from build123d import *

# Parameters (mm, degrees)
CROQUIS1_W               = 30
CROQUIS1_H               = 30
CROQUIS1_R               = 2.1
SALIENTE_EXTRUIR1_DEPTH  = 6
REDONDEO1_R              = 5
CROQUIS3_R               = 3.45
CORTAR_EXTRUIR2_DEPTH    = 2
REDONDEO1_OF_SIMETR_A1_R = 5
CROQUIS2_OUTSIDE_W       = 79.012
CROQUIS2_OUTSIDE_H       = 79.012
CROQUIS2_OUTSIDE_R       = 29
CORTAR_EXTRUIR1_DEPTH    = 3
CHAFL_N1_SIZE            = 0.5


with BuildPart() as part:
    # Croquis1 → Saliente-Extruir1 (new body)
    with BuildSketch(Plane(origin=(0, 0, 0), x_dir=(1, 0, 0), z_dir=(0, 1, 0))):
        with Locations((15, 15)):
            Rectangle(CROQUIS1_W, CROQUIS1_H)
        with Locations((25, 25)):
            Circle(CROQUIS1_R, mode=Mode.SUBTRACT)
        with BuildLine():
            Line((2.5, 3), (2.5, 25))
            ThreePointArc((2.5, 25), (4, 26.5), (5.5, 25))
            Line((5.5, 25), (5.5, 3))
            ThreePointArc((5.5, 3), (4, 1.5), (2.5, 3))
        make_face(mode=Mode.SUBTRACT)
        with BuildLine():
            Line((7.5, 3), (7.5, 25))
            ThreePointArc((7.5, 25), (9, 26.5), (10.5, 25))
            Line((10.5, 25), (10.5, 3))
            ThreePointArc((10.5, 3), (9, 1.5), (7.5, 3))
        make_face(mode=Mode.SUBTRACT)
        with BuildLine():
            Line((17.5, 3), (17.5, 25))
            ThreePointArc((17.5, 25), (19, 26.5), (20.5, 25))
            Line((20.5, 25), (20.5, 3))
            ThreePointArc((20.5, 3), (19, 1.5), (17.5, 3))
        make_face(mode=Mode.SUBTRACT)
        with BuildLine():
            Line((22.5, 3), (22.5, 19.36981464))
            ThreePointArc((22.5, 19.36981464), (24, 20.86981464), (25.5, 19.36981464))
            Line((25.5, 19.36981464), (25.5, 3))
            ThreePointArc((25.5, 3), (24, 1.5), (22.5, 3))
        make_face(mode=Mode.SUBTRACT)
        with BuildLine():
            Line((15.5, 25), (15.5, 3))
            ThreePointArc((15.5, 3), (14, 1.5), (12.5, 3))
            Line((12.5, 3), (12.5, 25))
            ThreePointArc((12.5, 25), (14, 26.5), (15.5, 25))
        make_face(mode=Mode.SUBTRACT)
    saliente_extruir1 = extrude(amount=SALIENTE_EXTRUIR1_DEPTH)

    # Redondeo1
    redondeo1_edges = [part.edges().sort_by_distance(p)[0] for p in [
        (30, 3, -30),
    ]]
    fillet(redondeo1_edges, radius=REDONDEO1_R)

    # Croquis3 → Cortar-Extruir2 (cut)
    with BuildSketch(Plane.XZ):
        with Locations((25, -25)):
            Circle(CROQUIS3_R)
    cortar_extruir2 = extrude(amount=-CORTAR_EXTRUIR2_DEPTH, mode=Mode.SUBTRACT)

    # Simetría1: Saliente-Extruir1, Cortar-Extruir2 across plane
    add(saliente_extruir1.mirror(Plane(origin=(0, 6, 0), x_dir=(1, 0, 0), z_dir=(0, 0, -1))))
    add(cortar_extruir2.mirror(Plane(origin=(0, 6, 0), x_dir=(1, 0, 0), z_dir=(0, 0, -1))), mode=Mode.SUBTRACT)

    # Redondeo1 of Simetría1
    redondeo1_of_simetr_a1_edges = [part.edges().sort_by_distance(p)[0] for p in [
        (30, 3, 30),
    ]]
    fillet(redondeo1_of_simetr_a1_edges, radius=REDONDEO1_OF_SIMETR_A1_R)

    # Simetría7: part across plane


with BuildPart() as part_1:
    add(part.part)
    add(part.part.mirror(Plane(origin=(0, 6, 0), x_dir=(0, 0, 1), z_dir=(1, 0, 0))))

    # Croquis2 outside → Cortar-Extruir1 (cut)
    with BuildSketch(Plane(origin=(0, 6, 0), x_dir=(1, 0, 0), z_dir=(0, 1, 0))):
        Rectangle(CROQUIS2_OUTSIDE_W, CROQUIS2_OUTSIDE_H)
        Circle(CROQUIS2_OUTSIDE_R, mode=Mode.SUBTRACT)
    extrude(amount=-CORTAR_EXTRUIR1_DEPTH, mode=Mode.SUBTRACT)

    # Chaflán1
    chafl_n1_edges = [part_1.edges().sort_by_distance(p)[0] for p in [
        (30, 0, 0),
        (0, 0, 30),
        (28.535533906, 0, 28.535533906),
        (-30, 0, 0),
        (-28.535533906, 0, -28.535533906),
        (-28.535533906, 0, 28.535533906),
        (0, 0, -30),
        (28.535533906, 0, -28.535533906),
    ]]
    chamfer(chafl_n1_edges, length=CHAFL_N1_SIZE)


solid = part_1.part
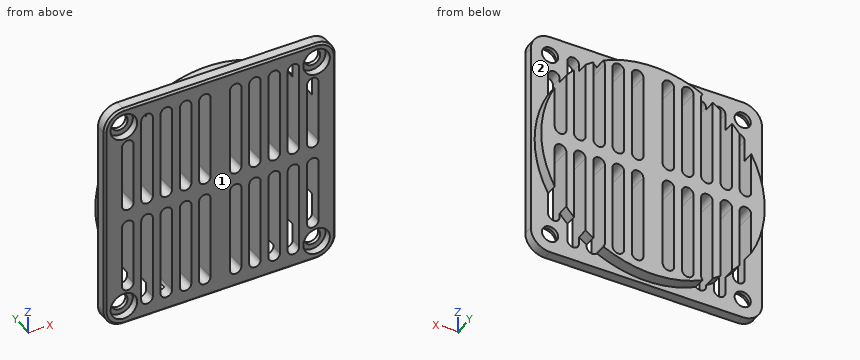
Source: CAD feature listing. Evaluate the final solid. Frame: model axes, mm. Face numbers are marked on the shaded views. A direction names the side the tool comes from. Give positions to 0.01 mm unless a question says otherwise; leave off trailing zeros. Write each loop counter-clockwise with the first axis right and the second up, starting at its lowest first coordinate (ties: lowest second). Pieces come first, ordered by that corner, then holes. Notation, with made-up numbers: M 79.5,-17.5 L 103.5,-17.5 A17 ccw 103.5,-8.5 Z; hole C -12,37 d6. An arc over 180 degrees is marked long. Return JSON: item names as keys, results as strings. Group by question number.
1) Pin query (flat end, axial travel): P1, Ø1, axis at x = -4.5, y = 4.5, coming from the -Z side; P2, Ø4, axis at x = -25, z = -25, coming from the -Y side; P3, Ø1.5, axis at x = -9.5, y = 4, coming from the -Z side; P4, Ø5, axis at x = 25, z = 25, coming from the +Y side. Return the tip coordinate at first contact, or that it passes through.
2) Cut plane A-A, the plane x = -14. Output: boundary loops of the cut face in (y, z).
3) Set-up query: the marked faces 1 and 2. Return all of +Z, -Z, +X, -X, +Y, -Y with unobstructed straight access to the full face (end or side cutting, diameter ignored); none if empty.
4) Cut plane B-B, the plane x = -24. Give the number of separate pieces and of enclosed holes in the cut face, plus the area to 3 significant figures.
5) Material intervals for line 1 along Z through (x, y) = (-4, 3.5); line 2 along Z through (x, y) = (13.5, 2); line 3 along Z through (x, y) = (25, 2.6), sorted ascending. Write a range as [from, to].
Recorded:
{
 "1": {"P1": "stops at z = -28.72", "P2": "passes through", "P3": "stops at z = -27.65", "P4": "stops at y = 3"},
 "2": {"outline": "M 0,-29.5 L 0.5,-30 L 3,-30 L 3,-26.5 L 0,-26.5 Z; M 0,-1.5 L 6,-1.5 L 6,1.5 L 0,1.5 Z; M 0,26.5 L 3,26.5 L 3,30 L 0.5,30 L 0,29.5 Z"},
 "3": {"face 1": "+Z, -Z, +X, -X, -Y", "face 2": "+Y"},
 "4": {"separate pieces": "5", "enclosed holes": "0", "area": "38.7 mm²"},
 "5": {"line 1": "z = [-28.72, -26.5], [-1.5, 1.5], [26.5, 28.72]", "line 2": "z = [-30, -26.41], [-1.59, 1.59], [26.41, 30]", "line 3": "z = [-30, -27.1], [-22.9, -20.49], [-1.88, 1.88], [20.49, 22.9], [27.1, 30]"}
}
